Check sheet for the modelled part. Datum: model origin and axes. Units: mm. A direction names the side the tool comes from. Give positions to 0.01 mm unless a question says otherwise; leave off trailing zeros. Order: outer loops, then holes, each group sorted by start corner. A loop starts at its lowest first (then second) coordinate and runs counter-clockwise, first axis right, second up. Notation, with made-up numbers: (18, 25) -> (72, 25) arc R15 cw to (72, 31) -> close; hole circle Ø9 at (2.25, 72). An arc over 180 degrees is marked (long way). Answer in a Markdown table with one row per item. Add a question column.
(1) Cross-section at A-A (z = 7.5). Record the cut outline in (x, y), then the cut area to 3 significant figures.
(2) Go/stop test with flat-tipped pins: pin 1 (6.5 mm diameter, centred on x = 6, z = 7.5, fed in from +Y); pin 2 (3 mm diameter, centred on y = 18.5, z = 7.5, fed in from +X); pin 3 (1 mm diameter, centred on x = -16.5, z = 158, fed in from -Y); pin 4 (2 mm diameter, centred on y = 19, z = 218, fed in from -X). Record where each tip stops, or that it passes through.
(3) Set-up check for faces 4 (the face through (52, 11.1, 15)), 5 (the face through (-48, 15, 15)), 6 (the face through (55, -8, 111)): record each of +Z, -Z, +X, -X, +Y, -Y from which the full face is reachable in a straight line by a thin tool's end or side.
(4) Cross-section at B-B (y = -10.5). Record the cut outline in (x, z).
(5) Cross-section at D-D (y = 9.5). Record the cut outline in (x, z).
(6) Thickness scan on L1, parallel to X at y = 19, z = 7; L2, parallel to X at y = -1.5, z = 193.5; L3, parallel to Y at x = 13, z = 123. Record the ranges inside material, lowest first. Write a range as [from, to].
(7) Cross-section at C-C (z = 112). Record the cut outline in (x, y), then the cut area to 3 significant figures.
(8) Release check for a two-part mould opening along X. For faces 1 (the face through (10.797, 18.768, 1.141)), 2 (the face through (6.751, 18.768, 9.885)), 3 (the face through (-10.797, 18.768, 223.859)) record: released by +X, released by -X, zero draft, split by the parting line, or undercut.
```python
from build123d import *

# Parameters (mm, degrees)
EXTRUDE_1_DEPTH     = 225
SHELL_2_T           = 2.5
SKETCH_2_R          = 2.5
CUT_EXTRUDE_1_DEPTH = 236.239239924


with BuildPart() as part:
    # 草图1 → 凸台-拉伸1 (new body)
    with BuildSketch(Plane.XY):
        with BuildLine():
            Line((-39, 17.5), (39, 17.5))
            ThreePointArc((39, 17.5), (50.313708499, 12.813708499), (55, 1.5))
            Line((55, 1.5), (55, -17.5))
            Line((55, -17.5), (-55, -17.5))
            Line((-55, -17.5), (-55, 1.5))
            ThreePointArc((-55, 1.5), (-50.313708499, 12.813708499), (-39, 17.5))
        make_face()
    extrude(amount=EXTRUDE_1_DEPTH)

    # 抽壳2
    shell_2_openings = [part.faces().sort_by_distance(p)[0] for p in [
        (0, -17.5, 112.5),
        (0, -0.40911681, 0),
        (0, -0.40911681, 225),
    ]]
    offset(amount=SHELL_2_T, openings=shell_2_openings, kind=Kind.INTERSECTION)

    # 草图2 → 切除-拉伸1 (cut, through all)
    with BuildSketch(Plane(origin=(0, 20, 0), x_dir=(1, 0, 0), z_dir=(0, 1, 0))):
        with Locations(Location((-6, -7.5, 0), (0, 0, 270))):
            Circle(SKETCH_2_R)
        with Locations(Location((6, -7.5, 0), (0, 0, 270))):
            Circle(SKETCH_2_R)
        with Locations(Location((6, -217.5, 0), (0, 0, 90))):
            Circle(SKETCH_2_R)
        with Locations(Location((-6, -217.5, 0), (0, 0, 90))):
            Circle(SKETCH_2_R)
        with BuildLine():
            Line((-8, 0), (-68.033168475, 0))
            Line((-68.033168475, 0), (-68.033168475, -15))
            Line((-68.033168475, -15), (-57.5, -15))
            Line((-57.5, -15), (-16, -15))
            ThreePointArc((-16, -15), (-13.171572875, -13.828427125), (-12, -11))
            Line((-12, -11), (-12, -4))
            ThreePointArc((-12, -4), (-10.828427125, -1.171572875), (-8, 0))
        make_face()
        with BuildLine():
            Line((68.316175474, -15), (68.316175474, 0))
            Line((68.316175474, 0), (8, 0))
            ThreePointArc((8, 0), (10.828427125, -1.171572875), (12, -4))
            Line((12, -4), (12, -11))
            ThreePointArc((12, -11), (13.171572875, -13.828427125), (16, -15))
            Line((16, -15), (68.316175474, -15))
        make_face()
        with BuildLine():
            Line((8, -225), (68.316175474, -225))
            Line((68.316175474, -225), (68.316175474, -210))
            Line((68.316175474, -210), (16, -210))
            ThreePointArc((16, -210), (13.171572875, -211.171572875), (12, -214))
            Line((12, -214), (12, -221))
            ThreePointArc((12, -221), (10.828427125, -223.828427125), (8, -225))
        make_face()
        with BuildLine():
            Line((-16, -210), (-57.5, -210))
            Line((-57.5, -210), (-68.033168475, -210))
            Line((-68.033168475, -210), (-68.033168475, -225))
            Line((-68.033168475, -225), (-8, -225))
            ThreePointArc((-8, -225), (-10.828427125, -223.828427125), (-12, -221))
            Line((-12, -221), (-12, -214))
            ThreePointArc((-12, -214), (-13.171572875, -211.171572875), (-16, -210))
        make_face()
    extrude(amount=-CUT_EXTRUDE_1_DEPTH, mode=Mode.SUBTRACT)


solid = part.part
```
Answer below:
| question | item | result |
|---|---|---|
| 1 | outline | (-12, 17.5) -> (-8.5, 17.5) -> (-8.5, 20) -> (-12, 20) -> close; (-3.5, 17.5) -> (3.5, 17.5) -> (3.5, 20) -> (-3.5, 20) -> close; (8.5, 17.5) -> (12, 17.5) -> (12, 20) -> (8.5, 20) -> close |
| 1 | area | 35.0 mm² |
| 2 | pin 1 | stops at y = 20 |
| 2 | pin 2 | stops at x = 12 |
| 2 | pin 3 | stops at y = 17.5 |
| 2 | pin 4 | stops at x = -12 |
| 3 | face 4 | -Z, +X, +Y, -Y |
| 3 | face 5 | -Z, -X, +Y, -Y |
| 3 | face 6 | +Z, -Z, -Y |
| 4 | outline | (-57.5, 15) -> (-55, 15) -> (-55, 210) -> (-57.5, 210) -> close; (55, 15) -> (57.5, 15) -> (57.5, 210) -> (55, 210) -> close |
| 5 | outline | (-55.68, 15) -> (-52.86, 15) -> (-52.86, 210) -> (-55.68, 210) -> close; (52.86, 15) -> (55.68, 15) -> (55.68, 210) -> (52.86, 210) -> close |
| 6 | L1 | x = [-12, -8.45], [-3.55, 3.55], [8.45, 12] |
| 6 | L2 | x = [-57.5, -55], [55, 57.5] |
| 6 | L3 | y = [17.5, 20] |
| 7 | outline | (-57.5, -17.5) -> (-55, -17.5) -> (-55, 1.5) arc R16 cw to (-39, 17.5) -> (39, 17.5) arc R16 cw to (55, 1.5) -> (55, -17.5) -> (57.5, -17.5) -> (57.5, 1.5) arc R18.5 ccw to (39, 20) -> (-39, 20) arc R18.5 ccw to (-57.5, 1.5) -> close |
| 7 | area | 425 mm² |
| 8 | face 1 | released by +X |
| 8 | face 2 | undercut |
| 8 | face 3 | released by -X |
